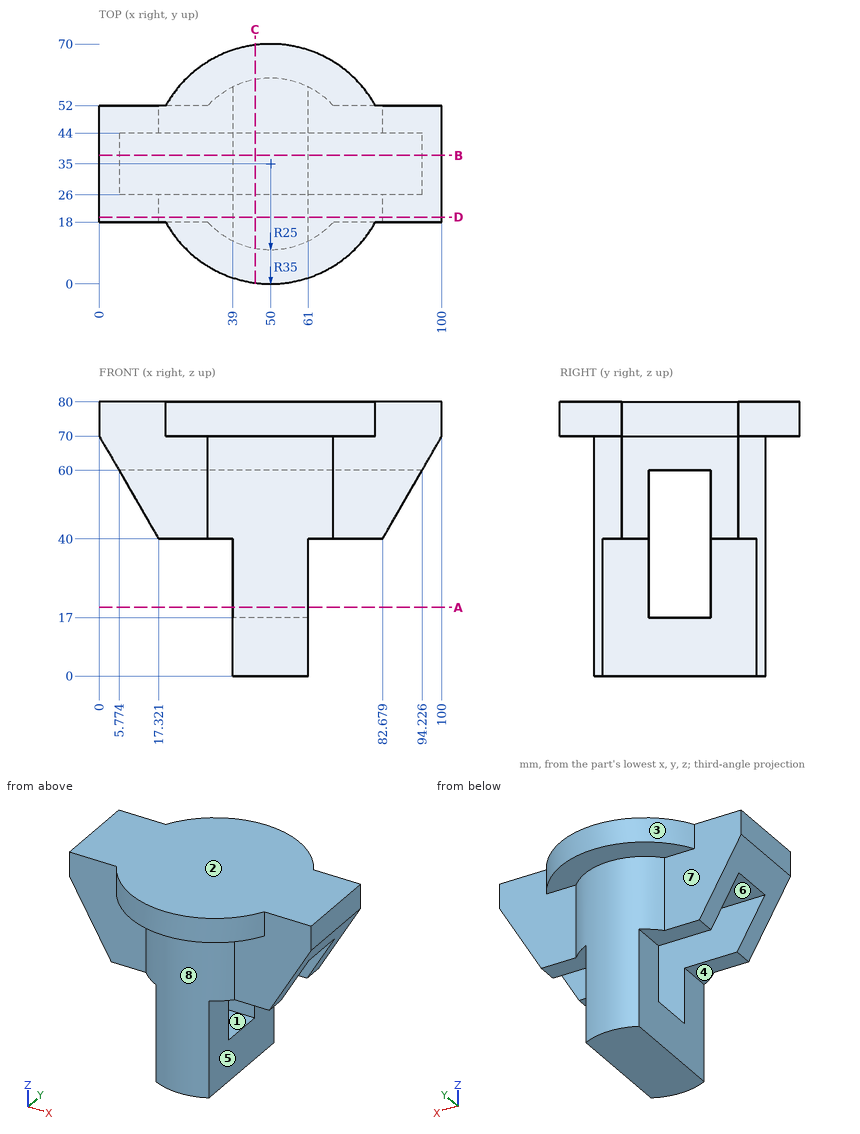
Print and shaded views of the part. All mm, measured from the part's lowest x, y and z. A direction names the side the tool comes from. Give positions to 0.01 mm unless a question says otherwise; leave off trailing zeros. Write each loop counter-clockwise with the first axis right and the second up, starting at its lowest first coordinate (ties: lowest second). Pieces come first, ordered by that corner, then holes. Notation, with made-up numbers: M 24.25,66 L 54.25,66 A28 cw 54.25,85 Z; hole C -7.75,70.25 d3. An arc over 180 degrees is marked long. Use a Markdown table: item, result.
1) Pin check, flat tips, straight feed: pin 1 (4 mm diameter, centred on y = 39, z = 61, fed in from -X); pin 2 (11 mm diameter, centred on x = 74, y = 54, fed in from -Z); pin 3 (6 mm diameter, centred on y = 37.5, z = 10.5, fed in from -X). Stop position of each tip, or through.
Responses:
| item | result |
|---|---|
| pin 1 | stops at x = 4.04 |
| pin 2 | stops at z = 40 |
| pin 3 | stops at x = 39 |
2) Cut at D-D (y = 19.5). List the corners of the cut face in (x, z).
Responses:
| item | result |
|---|---|
| outline | M 0,70 L 17.32,40 L 39,40 L 39,0 L 61,0 L 61,40 L 82.68,40 L 100,70 L 100,80 L 0,80 Z |
3) Pull direction Z, two halves, no side cores. Call the marked faces 1, 2 and 3: +Z half, -Z half, draft (parallel to the pull), parting line (faces both ways), or undercut.
Responses:
| item | result |
|---|---|
| face 1 | undercut |
| face 2 | +Z half |
| face 3 | draft |
4) Drill centre lines: line 1 (Z direction, x = 50.5, y = 36); line 2 (Y direction, x = 16.5, z = 64); line 3 (Z direction, x = 68, y = 33.5). Where is each one in solid material? Low to high. Write a range as from..to.
Responses:
| item | result |
|---|---|
| line 1 | z = 0..17, 60..80 |
| line 2 | y = 18..52 |
| line 3 | z = 60..80 |
5) Cut at A-A (z = 20). List the corners of the cut face in (x, y).
Responses:
| item | result |
|---|---|
| outline | M 39,12.55 A25 ccw 61,12.55 L 61,26 L 39,26 Z; M 39,44 L 61,44 L 61,57.45 A25 ccw 39,57.45 Z |
6) Cut at C-C (x = 45.5). List the corners of the cut face in (y, z), and give its area (3 significant figures).
Responses:
| item | result |
|---|---|
| outline | M 0.29,70 L 10.41,70 L 10.41,0 L 59.59,0 L 59.59,70 L 69.71,70 L 69.71,80 L 0.29,80 Z; hole M 26,17 L 44,17 L 44,60 L 26,60 Z |
| area | 3,360 mm2 |
7) Tool access for the marked faces 4, 5, 6, 7 and 8: list every direction of +Z, -Z, +X, -X, +Y, -Y with a clear straight run to the whole face (end or side of a thin tool).
Responses:
| item | result |
|---|---|
| face 4 | -Z, -X, +Y, -Y |
| face 5 | -Z, +X, +Y, -Y |
| face 6 | +X, -X |
| face 7 | -Z, -X, +Y |
| face 8 | -Z, -Y |
8) Cut at B-B (y = 37.5). List the corners of the cut face in (x, z), and give its area (3 significant figures).
Responses:
| item | result |
|---|---|
| outline | M 0,70 L 5.77,60 L 94.23,60 L 100,70 L 100,80 L 0,80 Z; M 39,0 L 61,0 L 61,17 L 39,17 Z |
| area | 2,320 mm2 |
